Part model, mm, in its own coordinate system. A direction names the side the tool comes from. Coordinates: 2 decimals unless noted, no trailing zeros. Order: outer loops, then holes, each group sorted by start corner. A loop starts at its lowest first (then second) coordinate and runs counter-clockwise, first axis right, second up.
from build123d import *

# Parameters (mm, degrees)
R_VOLUTION1_ANGLE       = 180
ENL_V_START             = -19
ESQUISSE2_W             = 120
ESQUISSE2_H             = 50.1
ENL_V_MAT_EXTRU_1_DEPTH = 10
ESQUISSE3_W             = 146.438377439
ESQUISSE3_H             = 50.311635948
ENL_V_MAT_EXTRU_2_DEPTH = 10
ESQUISSE4_W             = 156.060048108
ESQUISSE4_H             = 43.154210134
ENL_V_MAT_EXTRU_3_DEPTH = 7
CONG_1_R                = 10
ENL_V_MAT_EXTRU_4_DEPTH = 121
ESQUISSE6_R             = 1.4
ENL_V_MAT_EXTRU_5_DEPTH = 20


with BuildPart() as part:
    # Esquisse1 → Révolution1 (revolve, symmetric)
    with BuildSketch(Plane.XY) as r_volution1_sk:
        Polygon((70.5, -15.05), (99, -15.05), (99, -14.55), (100.5, -14.55), (100.5, -15.05), (100.5, -16.35), (103, -16.35), (103, -15.05), (114, -15.05), (114, -14.55), (115.5, -14.55), (115.5, -15.05), (115.5, -16.35), (118, -16.35), (118, -15.05), (120, -15.05), (120, -25.05), (0, -25.05), (0, -15.05), (0, -9.55), (70.5, -9.55), align=None)
    revolve(axis=Axis((0, 0, 0), (1, 0, 0)), revolution_arc=R_VOLUTION1_ANGLE / 2)
    revolve(r_volution1_sk.sketch, axis=Axis((0, 0, 0), (-1, 0, 0)), revolution_arc=R_VOLUTION1_ANGLE / 2)

    # Esquisse2 → Enlèv. mat.-Extru.1 (cut)
    with BuildSketch(Plane(origin=(0, 0, 0), x_dir=(1, 0, 0), z_dir=(0, 1, 0)).offset(ENL_V_START)):
        with Locations((60, 0)):
            Rectangle(ESQUISSE2_W, ESQUISSE2_H)
    extrude(amount=-ENL_V_MAT_EXTRU_1_DEPTH, mode=Mode.SUBTRACT)

    # Esquisse3 → Enlèv. mat.-Extru.2 (cut)
    with BuildSketch(Plane.XY.offset(ENL_V_START)):
        with Locations((56.62202011, -13.21090671)):
            Rectangle(ESQUISSE3_W, ESQUISSE3_H)
    enl_v_mat_extru_2 = extrude(amount=-ENL_V_MAT_EXTRU_2_DEPTH, mode=Mode.SUBTRACT)

    # Esquisse4 → Enlèv. mat.-Extru.3 (cut)
    with BuildSketch(Plane(origin=(0, -16.324904288, -19), x_dir=(-1, 0, 0), z_dir=(0, -0.651692786, -0.758483034))):
        with Locations((-53.986796091, -2.160595236)):
            Rectangle(ESQUISSE4_W, ESQUISSE4_H)
    enl_v_mat_extru_3 = extrude(amount=-ENL_V_MAT_EXTRU_3_DEPTH, mode=Mode.SUBTRACT)

    # Symétrie1: Enlèv. mat.-Extru.2, Enlèv. mat.-Extru.3 across plane
    add(enl_v_mat_extru_2.mirror(Plane.XY), mode=Mode.SUBTRACT)
    add(enl_v_mat_extru_3.mirror(Plane.XY), mode=Mode.SUBTRACT)

    # Congé1
    cong_1_edges = [part.edges().sort_by_distance(p)[0] for p in [
        (60, -5.583646825, 19),
        (60, -5.583646825, -19),
    ]]
    fillet(cong_1_edges, radius=CONG_1_R)

    # Esquisse5 → Enlèv. mat.-Extru.4 (cut, through all)
    with BuildSketch(Plane.ZY):
        Polygon((10.25, 0), (-10.25, 0), (-10.25, -9.9), (-3, -9.9), (-3, -13.9), (3, -13.9), (3, -9.9), (10.25, -9.9), align=None)
    extrude(amount=-ENL_V_MAT_EXTRU_4_DEPTH, mode=Mode.SUBTRACT)

    # Esquisse6 → Enlèv. mat.-Extru.5 (cut, through all)
    with BuildSketch(Plane(origin=(0, 0, 0), x_dir=(1, 0, 0), z_dir=(0, 1, 0))):
        with Locations((6.5, 14.625)):
            Circle(ESQUISSE6_R)
        with Locations((64, 14.625)):
            Circle(ESQUISSE6_R)
    enl_v_mat_extru_5 = extrude(amount=-ENL_V_MAT_EXTRU_5_DEPTH, mode=Mode.SUBTRACT)

    # Symétrie2: Enlèv. mat.-Extru.5 across plane
    add(enl_v_mat_extru_5.mirror(Plane.XY), mode=Mode.SUBTRACT)


solid = part.part
Q1. Wall check: line 1 along Z through (x, y) = (64, -5.75) (3 decimals); line 2 along X through (y, z) = (-0.75, -14); line 3 along X through (y, z) = (-10, -10). Give the ranges that are in metal, low to high.
Results list:
line 1: z = -18.22 to -16.025, -13.225 to -10.25, 10.25 to 13.225, 16.025 to 18.22
line 2: x = 0 to 5.25, 7.75 to 62.75, 65.25 to 70.5
line 3: x = 0 to 70.5
Q2. Cut at A-A on z = 0. Write the cut outline in (x, y), and give its area (3 significant figures).
Results list:
outline: (0, -19) - (120, -19) - (120, -15.05) - (118, -15.05) - (118, -16.35) - (115.5, -16.35) - (115.5, -14.55) - (114, -14.55) - (114, -15.05) - (103, -15.05) - (103, -16.35) - (100.5, -16.35) - (100.5, -14.55) - (99, -14.55) - (99, -15.05) - (70.5, -15.05) - (70.5, -13.9) - (0, -13.9) - close
area: 550 mm2
Q3. Cut at D-D on x = 94. Write the cut outline in (y, z), and give its area (3 significant figures).
Results list:
outline: (-19, -7.47) - (-8.39, -16.58) arc R10 ccw to (-1.88, -19) - (0, -19) - (0, -15.05) arc R15.05 cw to (0, 15.05) - (0, 19) - (-1.88, 19) arc R10 ccw to (-8.39, 16.58) - (-19, 7.47) - close
area: 208 mm2
Q4. Pin check, flat tips, straight feed: pin 1 Ø4.5 at (x, y) = (24.5, -11) entering from +Z; pin 2 Ø5 at (x, z) = (18.5, 1) entering from +Y; pin 3 Ø3 at (x, y) = (50.5, -11.5) entering from -Z. Stop position of each tip, or through.
Results list:
pin 1: stops at z = 16.28
pin 2: stops at y = -9.9
pin 3: stops at z = -15.21
Q5. Which spindle directions (+Z, -Z, +X, -X, +Y, -Y) get a long thin tool onto all of the face, cutting with end or side? Do faces 5 (the face through (63.697, -6.066, -13.258)), 6 (the face through (103, -15.4, 0.1)), 7 (the face through (60.84, -5.306, -18.394)), 8 (the face through (114.76, -14.546, -0.32)), 9 (the face through (35, -5, -10.25)). Say none if no direction does.
Results list:
face 5: +Y, -Y
face 6: +Y
face 7: -Z, +X, -X, -Y
face 8: +X, +Y
face 9: +X, -X, +Y
Q6. Cut at B-B on y = -5.5. Count the separate pieces of the cut face and the enclosed holes in it, and give its area (3 significant figures).
Results list:
separate pieces: 2
enclosed holes: 4
area: 1,530 mm2
Q7. Cut at C-C on x = 6.5. Write the cut outline in (y, z) (3 decimals).
Results list:
outline: (-19, -7.473) - (-12.305, -13.225) - (0, -13.225) - (0, -10.25) - (-9.9, -10.25) - (-9.9, -3) - (-13.9, -3) - (-13.9, 3) - (-9.9, 3) - (-9.9, 10.25) - (0, 10.25) - (0, 13.225) - (-12.305, 13.225) - (-19, 7.473) - close; (-9.046, -16.025) - (-8.395, -16.585) arc R10 ccw to (-1.878, -19) - (0, -19) - (0, -16.025) - close; (-9.046, 16.025) - (0, 16.025) - (0, 19) - (-1.878, 19) arc R10 ccw to (-8.395, 16.585) - close
Q8. Mould opens along Z. For faces 1 (the face through (63.697, -4.714, 13.258)), 2 (the face through (35, -9.9, 7)), 3 (the face through (0, -12, -4)), 4 (the face through (59.16, -5.306, 18.394)) say: pulls with the +Z half, pulls with the -Z half, needs draft (parallel to the pull), parting line crosses it, or undercut.
Results list:
face 1: undercut
face 2: undercut
face 3: needs draft
face 4: pulls with the +Z half
